Verification items for the finished model (mm, model axes). Face numbers are marked on the shaded views. A direction names the side the tool comes from. Give positions to 0.01 mm unless a question says otherwise; leave off trailing zeros. Write each loop counter-clockwise with the first axis right and the second up, starting at its lowest first coordinate (ties: lowest second). Pieces come first, ordered by that corner, then holes.
from build123d import *

# Parameters (mm, degrees)
SKETCH_1_W      = 35
SKETCH_1_H      = 17
EXTRUDE_1_DEPTH = 3
SKETCH_2_R      = 0.6
SKETCH_2_R_2    = 0.55
EXTRUDE_2_DEPTH = 3
FILLET_1_R      = 0.5


with BuildPart() as part:
    # 스케치1 → 보스-돌출1 (new body)
    with BuildSketch(Plane.XY):
        Rectangle(SKETCH_1_W, SKETCH_1_H)
        with BuildLine():
            Line((7.820550528, -4.5), (-7.820550528, -4.5))
            ThreePointArc((-7.820550528, -4.5), (-15, 0), (-7.820550528, 4.5))
            Line((-7.820550528, 4.5), (7.820550528, 4.5))
            ThreePointArc((7.820550528, 4.5), (12.655442773, 4.236581603), (15, 0))
            ThreePointArc((15, 0), (12.655442773, -4.236581603), (7.820550528, -4.5))
        make_face(mode=Mode.SUBTRACT)
    extrude(amount=EXTRUDE_1_DEPTH)

    # 스케치2 → 보스-돌출2 (add)
    with BuildSketch(Plane.XY.offset(3)):
        with Locations((-7.220550528, 4.5)):
            Circle(SKETCH_2_R)
        with Locations((-7.220550528, -4.5)):
            Circle(SKETCH_2_R)
        with Locations((7.270550528, -4.5)):
            Circle(SKETCH_2_R_2)
        with Locations((7.270550528, 4.5)):
            Circle(SKETCH_2_R_2)
    extrude(amount=-EXTRUDE_2_DEPTH)

    # 필렛1
    fillet_1_edges = [part.edges().sort_by_distance(p)[0] for p in [
        (-6.620550528, 4.5, 1.5),
        (-6.620550528, -4.5, 1.5),
        (6.720550528, -4.5, 1.5),
        (6.720550528, 4.5, 1.5),
    ]]
    fillet(fillet_1_edges, radius=FILLET_1_R)


solid = part.part
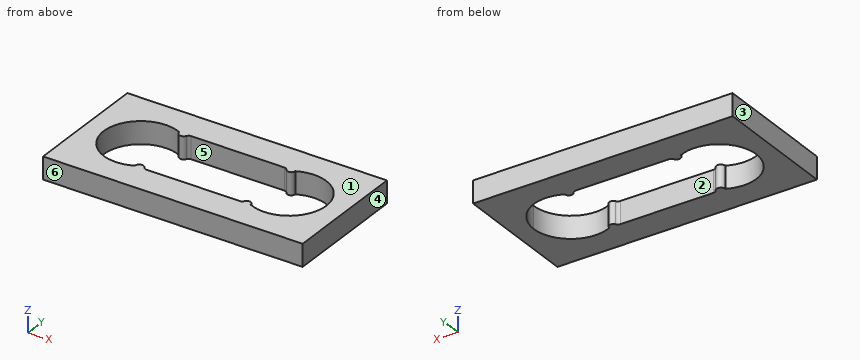
Item 1: Release check for a two-part mould opening along X. For the marked faces 3, 4, 5 and 6 record: released by +X, released by -X, zero draft, split by the parting line, or undercut.
Answer key:
face 3: released by -X
face 4: released by +X
face 5: undercut
face 6: zero draft
Item 2: Sectioned sample at C-C on y = -1.5. Record the cut outline in (x, z).
Answer key:
outline: (-17.5, 0) - (-14.77, 0) - (-14.77, 3) - (-17.5, 3) - close; (14.77, 0) - (17.5, 0) - (17.5, 3) - (14.77, 3) - close
Item 3: Depth check by flat-ended pin: pin 1 (8 mm diameter, centred on x = -10, y = 0, fed in from +Z). Enter the tip coordinate at first touch or a pass-through.
Answer key:
pin 1: passes through
Item 4: Scan lines: line 1 along X through (y, z) = (0, 0.9); line 2 along Y through (x, z) = (0.5, 0.5); line 3 along Y through (x, z) = (-10, 1.9). Record each from-to range of solid material in increasing order.
Answer key:
line 1: x = -17.5 to -15, 15 to 17.5
line 2: y = -8.5 to -4.5, 4.5 to 8.5
line 3: y = -8.5 to -5, 5 to 8.5
Item 5: Sectioned sample at A-A on x = -10. Record the cut outline in (y, z).
Answer key:
outline: (-8.5, 0) - (-5, 0) - (-5, 3) - (-8.5, 3) - close; (5, 0) - (8.5, 0) - (8.5, 3) - (5, 3) - close
Item 6: Sectioned sample at B-B on z = 1.9. Record the cut outline in (x, y).
Answer key:
outline: (-17.5, -8.5) - (17.5, -8.5) - (17.5, 8.5) - (-17.5, 8.5) - close; hole (-7.82, -4.5) arc R0.6 cw to (-6.69, -4.23) arc R0.5 ccw to (-6.24, -4.5) - (6.35, -4.5) arc R0.5 ccw to (6.79, -4.24) arc R0.55 cw to (7.82, -4.5) arc R5 ccw (long way) to (7.82, 4.5) arc R0.55 cw to (6.79, 4.24) arc R0.5 ccw to (6.35, 4.5) - (-6.24, 4.5) arc R0.5 ccw to (-6.69, 4.23) arc R0.6 cw to (-7.82, 4.5) arc R5 ccw (long way) to start
Item 7: Set-up check for the marked faces 1 and 2: record each of +Z, -Z, +X, -X, +Y, -Y from which the full face is reachable in a straight line by a thin tool's end or side.
Answer key:
face 1: +Z, +X, -X, +Y, -Y
face 2: +Z, -Z
